Can you work these out from the drawing? Everything is in mm from the part's minimum corner. Round coordinates to 2 decimals unless told otherwise and drop trailing zeros. Loops run counter-clockwise (first coordinate to the right, second up) from the corner with the lowest first, then second, coordinate; pieces in that order, holes last. Notation, with made-up numbers: M 79,-26.75 L 127,-26.75 A24 ccw 127,-0.75 Z; hole C 65,4.25 d3. An arc over 180 degrees is marked long. Use a Markdown table: item, result.
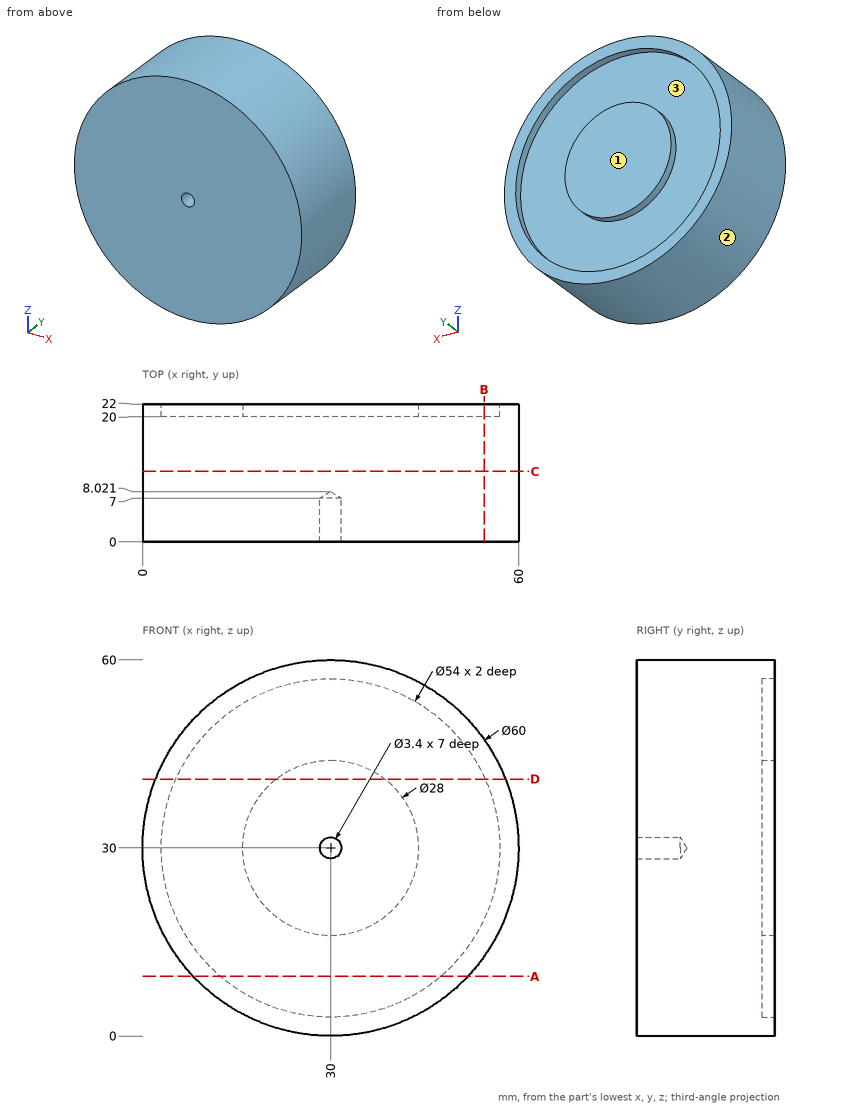
Q1. Imagine slicing it at A-A, the plane z = 9.5. Please give me the cut outline in (x, y).
Return value:
| item | result |
|---|---|
| outline | M 8.1,0 L 51.9,0 L 51.9,22 L 47.57,22 L 47.57,20 L 12.43,20 L 12.43,22 L 8.1,22 Z |
Q2. Will these pins go through, and if not, where does the flat tip stop? P1, Ø3, axis at x = 43.5, y = 8, coming from the -Z side (1 decimal); P2, Ø4, axis at x = 32.5, y = 12.5, coming from the -Z side; P3, Ø3, axis at y = 8, z = 32.5, coming from the +X side.
Return value:
| item | result |
|---|---|
| P1 | stops at z = 2.5 |
| P2 | stops at z = 0 |
| P3 | stops at x = 59.98 |
Q3. We'd pull the mould along Z, two halves only. Please class the marked faces 1, 2 and 3: pulls with the +Z half, pulls with the -Z half, needs draft (parallel to the pull), parting line crosses it, or undercut.
Return value:
| item | result |
|---|---|
| face 1 | needs draft |
| face 2 | parting line crosses it |
| face 3 | undercut |
Q4. I need wall thicknesses on line 1 (X direction, y = 21.45, z = 30); line 2 (X direction, y = 5, z = 30); line 3 (X direction, y = 21.25, z = 25.5). Which ranges of each line are inside material? Lowest first, please. Write a range as from..to.
Return value:
| item | result |
|---|---|
| line 1 | x = 0..3, 16..44, 57..60 |
| line 2 | x = 0..28.3, 31.7..60 |
| line 3 | x = 0.34..3.38, 16.74..43.26, 56.62..59.66 |
Q5. Imagine slicing it at D-D, the plane z = 41. Please give me the cut outline in (x, y).
Return value:
| item | result |
|---|---|
| outline | M 2.09,0 L 57.91,0 L 57.91,22 L 54.66,22 L 54.66,20 L 38.66,20 L 38.66,22 L 21.34,22 L 21.34,20 L 5.34,20 L 5.34,22 L 2.09,22 Z |
Q6. Imagine slicing it at C-C, the plane y = 11.25. Please give me the cut outline in (x, z).
Return value:
| item | result |
|---|---|
| outline | C 30,30 d60 |
Q7. Imagine slicing it at B-B, the plane x = 54.5. Please give me the cut outline in (y, z).
Return value:
| item | result |
|---|---|
| outline | M 0,12.69 L 22,12.69 L 22,18.65 L 20,18.65 L 20,41.35 L 22,41.35 L 22,47.31 L 0,47.31 Z |
